The listing builds one solid part. Answer for the finished solid, in the listing's coordinates (mm). Face numbers are marked on the shaded views. A direction names the side the tool comes from. Give positions to 0.01 mm unless a question says otherwise; leave off trailing zeros. Order: outer loops, then holes, each group sorted by start corner. A loop starts at its lowest first (then second) coordinate and runs counter-clockwise, first axis right, second up.
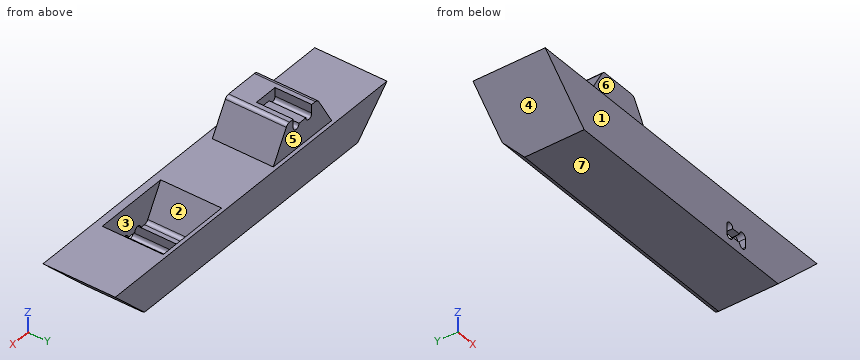
```python
from build123d import *

# Parameters (mm, degrees)
SKETCH1_W           = 139.7
SKETCH1_H           = 20
BOSS_EXTRUDE1_DEPTH = 14.17
CUT_EXTRUDE1_DEPTH  = 23.9
BOSS_EXTRUDE2_DEPTH = 23.9
CHAMFER1_SIZE       = 20
CHAMFER2_SIZE       = 5
CUT_EXTRUDE2_DEPTH  = 14.41
CUT_EXTRUDE3_DEPTH  = 19.02
FILLET1_R           = 2


with BuildPart() as part:
    # Sketch1 → Boss-Extrude1 (new, symmetric)
    with BuildSketch(Plane(origin=(0, 0, 0), x_dir=(1, 0, 0), z_dir=(0, 1, 0))):
        Rectangle(SKETCH1_W, SKETCH1_H)
    extrude(amount=BOSS_EXTRUDE1_DEPTH, both=True)

    # Sketch3 → Cut-Extrude1 (cut)
    with BuildSketch(Plane(origin=(0, -11.17, 0), x_dir=(-1, 0, 0), z_dir=(0, -1, 0))):
        Polygon((-13.283333333, -10), (-20.500211698, 2.5), (-36.066454968, 2.5), (-43.283333333, -10), align=None)
    extrude(amount=-CUT_EXTRUDE1_DEPTH, mode=Mode.SUBTRACT)

    # Sketch4 → Boss-Extrude2 (add)
    with BuildSketch(Plane(origin=(0, -11.17, 0), x_dir=(-1, 0, 0), z_dir=(0, -1, 0))):
        Polygon((43.283333333, -10), (13.283333333, -10), (20.500211698, -22.5), (36.066454968, -22.5), align=None)
    extrude(amount=-BOSS_EXTRUDE2_DEPTH)

    # Chamfer1
    chamfer1_edges = [part.edges().sort_by_distance(p)[0] for p in [
        (69.85, 0, -10),
        (-69.85, 0, -10),
    ]]
    chamfer(chamfer1_edges, length=CHAMFER1_SIZE - 0.0001)  # a hair under: the kernel refuses the full size

    # Chamfer2
    chamfer2_edges = [part.edges().sort_by_distance(p)[0] for p in [
        (0, 14.17, -10),
    ]]
    chamfer(chamfer2_edges, length=CHAMFER2_SIZE)

    # Sketch5 → Cut-Extrude2 (cut)
    with BuildSketch(Plane(origin=(0, 12.73, 0), x_dir=(1, 0, 0), z_dir=(0, 1, 0))):
        with BuildLine():
            Line((-33.048333333, -19.12), (-33.048333333, -22.5))
            Line((-33.048333333, -22.5), (-23.518333333, -22.5))
            Line((-23.518333333, -22.5), (-23.518333333, -19.12))
            ThreePointArc((-23.518333333, -19.12), (-25.018333333, -17.62), (-26.518333333, -19.12))
            Line((-26.518333333, -19.12), (-30.048333333, -19.12))
            ThreePointArc((-30.048333333, -19.12), (-31.548333333, -17.62), (-33.048333333, -19.12))
        make_face()
    extrude(amount=-CUT_EXTRUDE2_DEPTH, mode=Mode.SUBTRACT)

    # Sketch7 → Cut-Extrude3 (cut)
    with BuildSketch(Plane.XZ.offset(14.17)):
        with BuildLine():
            Line((23.518333333, -2.5), (23.518333333, -5.88))
            ThreePointArc((23.518333333, -5.88), (25.018333333, -7.38), (26.518333333, -5.88))
            Line((26.518333333, -5.88), (30.048333333, -5.88))
            ThreePointArc((30.048333333, -5.88), (31.548333333, -7.38), (33.048333333, -5.88))
            Line((33.048333333, -5.88), (33.048333333, -2.5))
            ThreePointArc((33.048333333, -2.5), (31.548333333, -1), (30.048333333, -2.5))
            Line((30.048333333, -2.5), (26.518333333, -2.5))
            ThreePointArc((26.518333333, -2.5), (25.018333333, -1), (23.518333333, -2.5))
        make_face()
    extrude(amount=-CUT_EXTRUDE3_DEPTH, mode=Mode.SUBTRACT)

    # Fillet1
    fillet1_edges = [part.edges().sort_by_distance(p)[0] for p in [
        (36.066454968, 0.78, -2.5),
        (20.500211698, 0.78, -2.5),
        (-36.066454968, 0.78, 22.5),
        (-20.500211698, 0.78, 22.5),
    ]]
    fillet(fillet1_edges, radius=FILLET1_R)


solid = part.part
```
1) Find section C-C (x = 41). Write down the section's boundary in (y, z).
Geometry says:
outline: (-14.17, -10) - (9.17, -10) - (14.17, -5) - (14.17, 10) - (12.73, 10) - (12.73, 6.05) - (-11.17, 6.05) - (-11.17, 10) - (-14.17, 10) - close
2) For a pull along X with two mould halves and no side action, classify the marked faces 1, 2, 3 and 4 as +X half, -X half, draft (parallel to the pull), parting line (faces both ways), or undercut.
Geometry says:
face 1: draft
face 2: undercut
face 3: undercut
face 4: -X half
3) A tool of negligible diameter and unlimited length cuts with its end or side. For the marked faces 5, 6 and 7, from which of +Z, -Z, +X, -X, +Y, -Y can it reach the whole face along a straight path? Write none if from no direction.
Geometry says:
face 5: +Z, +X, -X, +Y
face 6: +Z, +X, -X, -Y
face 7: -Z, +X, -X, +Y, -Y
4) Given P1, Ø1.1, axis at x = -28.5, y = 9, coming from the +Z side; P2, Ø10, axis at x = -26.5, z = 19, coming from the +Y side; P3, Ø14, axis at x = -29.5, z = 18, coming from the -Y side, each flat-ended and moving along its own axis, determine where each tip first touches the part or whether it passes through.
Geometry says:
P1: stops at z = 19.12
P2: stops at y = 12.73
P3: stops at y = -11.17
5) Find section D-D (z = 16). Write down the section's boundary in (x, y), then the cut area to 3 significant figures.
Geometry says:
outline: (-39.82, -11.17) - (-16.75, -11.17) - (-16.75, 12.73) - (-39.82, 12.73) - close
area: 551 mm2
6) Straight lines are drawn through the part: probe 1 along Z at (x, y) = (-9.5, -2.75); probe 2 along X at (y, z) = (-8.25, 1); probe 3 along X at (y, z) = (-0.5, 20.5). For each, find the intervals that lie inside material, in ascending order.
Geometry says:
probe 1: z = -10 to 10
probe 2: x = -60.85 to 18.48, 38.09 to 60.85
probe 3: x = -37.22 to -33.05, -23.52 to -19.35
7) Find section A-A (z = 8.5). Write down the section's boundary in (x, y).
Geometry says:
outline: (-68.35, -14.17) - (68.35, -14.17) - (68.35, 14.17) - (-68.35, 14.17) - close; hole (14.15, -11.17) - (42.42, -11.17) - (42.42, 12.73) - (14.15, 12.73) - close
